from build123d import *

# Parameters (mm, degrees)
SKETCH_1_W          = 37
SKETCH_1_H          = 59
EXTRUDE_1_DEPTH     = 2
SKETCH_2_W          = 20
SKETCH_2_H          = 40
CUT_EXTRUDE_1_DEPTH = 2
SKETCH_3_W          = 2
SKETCH_3_H          = 59
EXTRUDE_2_DEPTH     = 31
SKETCH_4_W          = 2
SKETCH_4_H          = 59
EXTRUDE_3_DEPTH     = 20
SKETCH_5_R          = 2
CUT_EXTRUDE_2_DEPTH = 20
SKETCH_6_R          = 2.5
CUT_EXTRUDE_3_DEPTH = 20


with BuildPart() as part:
    # 草图1 → 凸台-拉伸1 (new body)
    with BuildSketch(Plane.XY):
        with Locations((18.5, 29.5)):
            Rectangle(SKETCH_1_W, SKETCH_1_H)
    extrude(amount=EXTRUDE_1_DEPTH)

    # 草图2 → 切除-拉伸1 (cut)
    with BuildSketch(Plane.XY.offset(2)):
        with Locations((27, 29.5)):
            Rectangle(SKETCH_2_W, SKETCH_2_H)
    extrude(amount=-CUT_EXTRUDE_1_DEPTH, mode=Mode.SUBTRACT)

    # 草图3 → 凸台-拉伸2 (add)
    with BuildSketch(Plane(origin=(0, 0, 0), x_dir=(-1, 0, 0), z_dir=(0, 0, -1))):
        with Locations((-1, 29.5)):
            Rectangle(SKETCH_3_W, SKETCH_3_H)
    extrude(amount=EXTRUDE_2_DEPTH)

    # 草图4 → 凸台-拉伸3 (add)
    with BuildSketch(Plane.ZY):
        with Locations((-30, 29.5)):
            Rectangle(SKETCH_4_W, SKETCH_4_H)
    extrude(amount=EXTRUDE_3_DEPTH)

    # 草图5 → 切除-拉伸2 (cut)
    with BuildSketch(Plane(origin=(0, 0, -31), x_dir=(-1, 0, 0), z_dir=(0, 0, -1))):
        with Locations((10, 44.5)):
            Circle(SKETCH_5_R)
        with Locations((10, 14.5)):
            Circle(SKETCH_5_R)
    extrude(amount=-CUT_EXTRUDE_2_DEPTH, mode=Mode.SUBTRACT)

    # 草图6 → 切除-拉伸3 (cut)
    with BuildSketch(Plane(origin=(0, 0, 0), x_dir=(-1, 0, 0), z_dir=(0, 0, -1))):
        with Locations((-32, 54.5)):
            Circle(SKETCH_6_R)
        with Locations((-19.5, 54.5)):
            Circle(SKETCH_6_R)
        with Locations((-19.5, 4.5)):
            Circle(SKETCH_6_R)
        with Locations((-32, 4.5)):
            Circle(SKETCH_6_R)
    extrude(amount=-CUT_EXTRUDE_3_DEPTH, mode=Mode.SUBTRACT)


solid = part.part
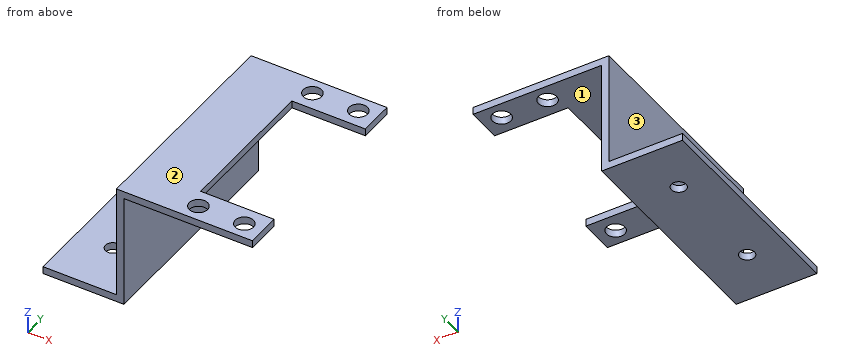
Here's how the part is built. I have some questions about the finished solid (model axes, mm). Face numbers are marked on the shaded views. A direction names the side the tool comes from. Give positions to 0.01 mm unless a question says otherwise; leave off trailing zeros. Order: outer loops, then holes, each group sorted by start corner. A loop starts at its lowest first (then second) coordinate and runs counter-clockwise, first axis right, second up. Notation, with made-up numbers: M 42.5,27.5 L 63.5,27.5 A24 cw 63.5,58.5 Z; hole C 1.5,-9.75 d6. An arc over 180 degrees is marked long. Answer as a JSON object with one key per item and string values. Group by question number.
1) Suppose I cut it at B-B, the plane x = 32. Write out the boundary of the cut face in (y, z), plus the area to 3 significant figures.
2) Suppose I cut it at C-C, the plane y = 4.5. Write out the boundary of the cut face in (x, z), plus the area to 3 significant figures.
3) On a 3-axis mill with a long thin cutter (end or side, diameter ignored), from which of +Z, -Z, +X, -X, +Y, -Y can I reach the whole of each face in a straight line? I mean the marked faces 1, 2 and 3. Say none if no direction works.
4) Suppose I cut it at D-D, the plane y = 27.5. Write out the boundary of the cut face in (x, z), plus the area to 3 significant figures.
5) I'm going to push flat-ended pins straight in: pin 1 Ø1 at (y, z) = (48.5, -23) entering from +X; pin 2 Ø17.5 at (x, y) = (16.5, 31.5) entering from -Z; pin 3 Ø15.5 at (y, z) = (21.5, -16) entering from -X. Where does each tip first touch, or does it pass through?
6) Suppose I cut it at A-A, the plane y = 14.5. Write out the boundary of the cut face in (x, z).
7) Please list where these lines run through material, in increasing order: L1, parallel to Y at x = 32, z = 1; L2, parallel to Y at x = -10, z = -30.05; L3, parallel to Y at x = 19, z = 1. Write a range as [from, to].
Results found:
{
 "1": {"outline": "M 0,0 L 2,0 L 2,2 L 0,2 Z; M 7,0 L 9.5,0 L 9.5,2 L 7,2 Z; M 49.5,0 L 52,0 L 52,2 L 49.5,2 Z; M 57,0 L 59,0 L 59,2 L 57,2 Z", "area": "18.0 mm²"},
 "2": {"outline": "M -20,-31 L 2,-31 L 2,0 L 17,0 L 17,2 L 0,2 L 0,-29 L -20,-29 Z; M 22,0 L 29.5,0 L 29.5,2 L 22,2 Z; M 34.5,0 L 37,0 L 37,2 L 34.5,2 Z", "area": "156 mm²"},
 "3": {"face 1": "-Z, +X, +Y, -Y", "face 2": "+Z, +X, -X, +Y, -Y", "face 3": "+Z, -X, +Y, -Y"},
 "4": {"outline": "M -20,-31 L 2,-31 L 2,0 L 17,0 L 17,2 L 0,2 L 0,-29 L -20,-29 Z", "area": "136 mm²"},
 "5": {"pin 1": "x = 2", "pin 2": "z = 0", "pin 3": "x = 0"},
 "6": {"outline": "M -20,-31 L -12,-31 L -12,-29 L -20,-29 Z; M -8,-31 L 2,-31 L 2,0 L 17,0 L 17,2 L 0,2 L 0,-29 L -8,-29 Z"},
 "7": {"L1": "[0, 2], [7, 9.5], [49.5, 52], [57, 59]", "L2": "[0, 12.5], [16.5, 42.5], [46.5, 59]", "L3": "[0, 2.05], [6.95, 9.5], [49.5, 52.05], [56.95, 59]"}
}
